Verification items for the finished model (mm, model axes). Give positions to 0.01 mm unless a question says otherwise; leave off trailing zeros. Order: outer loops, then holes, each group sorted by start corner. A loop starts at its lowest first (then second) coordinate and runs counter-clockwise, first axis right, second up. Notation, with made-up numbers: M 13.25,77 L 25.25,77 A17 cw 25.25,85 Z; hole C 75.5,52.25 d7. An arc over 180 degrees is marked long. Answer as a JSON object with one key per item and string values.
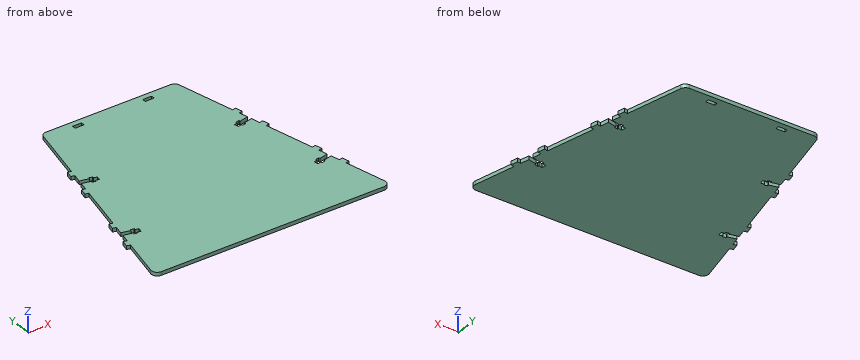
```python
from build123d import *

# Parameters (mm, degrees)
F0_W     = 7.9375
F0_H     = 3.175
F1_DEPTH = 3.175
F2_R     = 5.08


with BuildPart() as f1:
    # F0 (on Top) → F1 (new body)
    with BuildSketch(Plane.XY):
        Polygon((59.53125, 101.6), (-59.53125, 101.6), (-71.808473, 47.410876), (-74.904995, 48.112431), (-76.308106, 41.919389), (-73.211585, 41.217833), (-74.965474, 33.476529), (-67.22417, 31.72264), (-66.943548, 32.961249), (-63.847027, 32.259693), (-64.127649, 31.021085), (-61.031128, 30.319529), (-61.872994, 26.603703), (-64.969516, 27.305259), (-65.250138, 26.066651), (-68.346659, 26.768206), (-68.066037, 28.006815), (-75.807341, 29.760704), (-77.56123, 22.0194), (-80.657751, 22.720956), (-82.060862, 16.527913), (-78.964341, 15.826358), (-88.78612, -27.524942), (-91.882641, -26.823386), (-93.285752, -33.016429), (-90.189231, -33.717985), (-91.94312, -41.459288), (-84.201816, -43.213177), (-83.921194, -41.974569), (-80.824673, -42.676124), (-81.105295, -43.914733), (-78.008774, -44.616288), (-78.85064, -48.332114), (-81.947162, -47.630558), (-82.227784, -48.869167), (-85.324305, -48.167611), (-85.043683, -46.929003), (-92.784987, -45.175114), (-94.538876, -52.916417), (-97.635397, -52.214862), (-99.038508, -58.407904), (-95.941987, -59.10946), (-105.56875, -101.6), (105.56875, -101.6), (95.941987, -59.10946), (99.038508, -58.407904), (97.635397, -52.214862), (94.538876, -52.916417), (92.784987, -45.175114), (85.043683, -46.929003), (85.324305, -48.167611), (82.227784, -48.869167), (81.947162, -47.630558), (78.85064, -48.332114), (78.008774, -44.616288), (81.105295, -43.914733), (80.824673, -42.676124), (83.921194, -41.974569), (84.201816, -43.213177), (91.94312, -41.459288), (90.189231, -33.717985), (93.285752, -33.016429), (91.882641, -26.823386), (88.78612, -27.524942), (78.964341, 15.826358), (82.060862, 16.527913), (80.657751, 22.720956), (77.56123, 22.0194), (75.807341, 29.760704), (68.066037, 28.006815), (68.346659, 26.768206), (65.250138, 26.066651), (64.969516, 27.305259), (61.872994, 26.603703), (61.031128, 30.319529), (64.127649, 31.021085), (63.847027, 32.259693), (66.943548, 32.961249), (67.22417, 31.72264), (74.965474, 33.476529), (73.211585, 41.217833), (76.308106, 41.919389), (74.904995, 48.112431), (71.808473, 47.410876), align=None)
        with Locations((-31.241504, 95.25)):
            Rectangle(F0_W, F0_H, mode=Mode.SUBTRACT)
        with Locations((31.241504, 95.25)):
            Rectangle(F0_W, F0_H, mode=Mode.SUBTRACT)
    extrude(amount=F1_DEPTH)

    # F2
    f2_edges = [f1.edges().sort_by_distance(p)[0] for p in [
        (-59.53125, 101.6, 1.5875),
        (59.53125, 101.6, 1.5875),
        (105.56875, -101.6, 1.5875),
        (-105.56875, -101.6, 1.5875),
    ]]
    fillet(f2_edges, radius=F2_R)


solid = f1.part
```
Q1. Section check B-B on y = -0.5. Record the cut outline in (x, z) (3 decimals).
Resolved:
{"outline": "M -82.663,0 L 82.663,0 L 82.663,3.175 L -82.663,3.175 Z"}
Q2. Material ranges on L1, parallel to Y at x = -35, z = 1.7; L2, parallel to X at y = 23, z = 2.5; L3, parallel to Y at x = -72.5, z = 2.9, recorded low to high.
Resolved:
{"L1": "y = -101.6 to 93.66, 96.84 to 101.6", "L2": "x = -77.34 to 77.34", "L3": "y = -101.6 to 29.01, 32.92 to 47.57"}
Q3. Section check C-C on y = -86.5. Record the cut outline in (x, z) (3 decimals).
Resolved:
{"outline": "M -102.148,0 L 102.148,0 L 102.148,3.175 L -102.148,3.175 Z"}
Q4. Section check A-A on z = 0.6. Count the separate pieces of the cut face and the enclosed holes in it, then the cut area to 3 significant figures.
Resolved:
{"separate pieces": "1", "enclosed holes": "2", "area": "33,400 mm²"}
Q5. Gauge pin test, flat ends, axial feed: pin 1 Ø5 at (x, y) = (-51, 57.5) entering from -Z; pin 2 Ø1.6 at (y, z) = (94.5, 1.5) entering from -X. Record the tip position at first contact, or that the pin passes through.
Resolved:
{"pin 1": "stops at z = 0", "pin 2": "stops at x = -61.32"}
